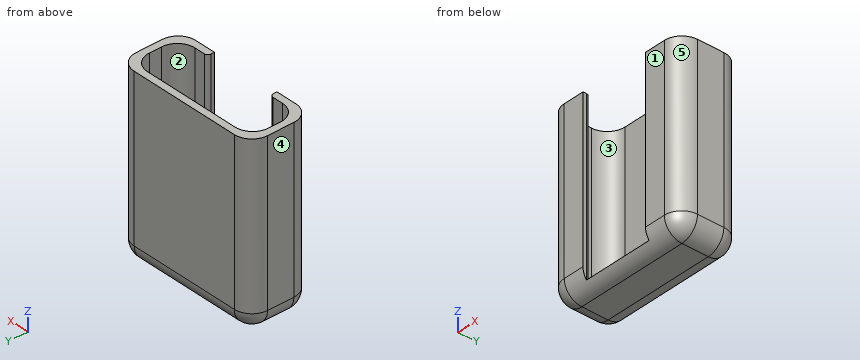
```python
from build123d import *

# Parameters (mm, degrees)
F1_DEPTH     = 50
F0_W         = 20
F0_H         = 2
F2_DEPTH     = 2
F3_T1_DEPTH  = 48
F3_T3_DEPTH  = 57.5
F3_T5_DEPTH  = 32
F3_T7_DEPTH  = 7.5
F3_S11_W     = 5
F3_S11_H     = 5
F3_T12_DEPTH = 5
F3_S17_W     = 5
F3_S17_H     = 5
F3_T18_DEPTH = 5
F3_S23_W     = 5
F3_S23_H     = 5
F3_T24_DEPTH = 5
F3_S29_W     = 5
F3_S29_H     = 5
F3_T30_DEPTH = 5
F4_R         = 1


# Not quite as in the source:
# - a fillet or chamfer that OpenCascade refuses, or shapes differently, is made with other operations: its cross-section is extruded or revolved along the edge and cut away or added


with BuildPart() as f1:
    # F0 (on Top) → F1 (new body)
    with BuildSketch(Plane.XY):
        Polygon((0, 0), (-9, 0), (-9, 13.5), (29, 13.5), (29, 0), (20, 0), (20, -2), (31, -2), (31, 15.5), (-11, 15.5), (-11, -2), (0, -2), align=None)
    extrude(amount=F1_DEPTH)

    # F0 (on Top) → F2 (join)
    with BuildSketch(Plane.XY):
        Polygon((-9, 13.5), (-9, 0), (0, 0), (20, 0), (29, 0), (29, 13.5), align=None)
        with Locations((10, -1)):
            Rectangle(F0_W, F0_H)
    extrude(amount=F2_DEPTH)

    # F3: fillet of radius 5 on 12 edges, made by hand

    # F3_s2 → F3_t1 (join)
    with BuildSketch(Plane.XY.offset(2)):
        with BuildLine():
            ThreePointArc((24, 0), (27.5355339059, 1.4644660941), (29, 5))
            Line((29, 5), (29, 0))
            Line((29, 0), (24, 0))
        make_face()
        with BuildLine():
            ThreePointArc((29, 8.5), (27.5355339059, 12.0355339059), (24, 13.5))
            Line((24, 13.5), (29, 13.5))
            Line((29, 13.5), (29, 8.5))
        make_face()
        with BuildLine():
            ThreePointArc((-4, 0), (-7.5355339059, 1.4644660941), (-9, 5))
            Line((-9, 5), (-9, 0))
            Line((-9, 0), (-4, 0))
        make_face()
        with BuildLine():
            ThreePointArc((-4, 13.5), (-7.5355339059, 12.0355339059), (-9, 8.5))
            Line((-9, 8.5), (-9, 13.5))
            Line((-9, 13.5), (-4, 13.5))
        make_face()
    extrude(amount=F3_T1_DEPTH)

    # F3_s4 → F3_t3 (cut)
    with BuildSketch(Plane.XY.offset(5)):
        with BuildLine():
            ThreePointArc((-6, 15.5), (-9.5355339059, 14.0355339059), (-11, 10.5))
            Line((-11, 10.5), (-11, 15.5))
            Line((-11, 15.5), (-6, 15.5))
        make_face()
        with BuildLine():
            ThreePointArc((-6, -2), (-9.5355339059, -0.5355339059), (-11, 3))
            Line((-11, 3), (-11, -2))
            Line((-11, -2), (-6, -2))
        make_face()
        with BuildLine():
            ThreePointArc((31, 10.5), (29.5355339059, 14.0355339059), (26, 15.5))
            Line((26, 15.5), (31, 15.5))
            Line((31, 15.5), (31, 10.5))
        make_face()
        with BuildLine():
            ThreePointArc((26, -2), (29.5355339059, -0.5355339059), (31, 3))
            Line((31, 3), (31, -2))
            Line((31, -2), (26, -2))
        make_face()
    extrude(amount=F3_T3_DEPTH, mode=Mode.SUBTRACT)

    # F3_s6 → F3_t5 (cut)
    with BuildSketch(Plane.YZ.offset(-6)):
        with BuildLine():
            ThreePointArc((-2, 5), (-0.5355339059, 1.4644660941), (3, 0))
            Line((3, 0), (-2, 0))
            Line((-2, 0), (-2, 5))
        make_face()
        with BuildLine():
            ThreePointArc((15.5, 5), (14.0355339059, 1.4644660941), (10.5, 0))
            Line((10.5, 0), (15.5, 0))
            Line((15.5, 0), (15.5, 5))
        make_face()
    extrude(amount=F3_T5_DEPTH, mode=Mode.SUBTRACT)

    # F3_s8 → F3_t7 (cut)
    with BuildSketch(Plane.XZ.offset(-10.5)):
        with BuildLine():
            ThreePointArc((31, 5), (29.5355339059, 1.4644660941), (26, 0))
            Line((26, 0), (31, 0))
            Line((31, 0), (31, 5))
        make_face()
        with BuildLine():
            ThreePointArc((-11, 5), (-9.5355339059, 1.4644660941), (-6, 0))
            Line((-6, 0), (-11, 0))
            Line((-11, 0), (-11, 5))
        make_face()
    extrude(amount=F3_T7_DEPTH, mode=Mode.SUBTRACT)


with BuildPart() as f3_tool10:
    # F3_s11 → F3_t12 (new body)
    with BuildSketch(Plane.XY.offset(5)):
        with Locations((-8.5, 13)):
            Rectangle(F3_S11_W, F3_S11_H)
    extrude(amount=-F3_T12_DEPTH)

    # F3_s13 → F3_t14 (revolve, cut)
    with BuildSketch(Plane(origin=(-6, 10.5, 5), x_dir=(0.7071067812, -0.7071067812, 0), z_dir=(0.7071067812, 0.7071067812, 0))):
        with BuildLine():
            ThreePointArc((0, -5), (5, 0), (0, 5))
            Line((0, 5), (0, -5))
        make_face()
    revolve(axis=Axis((-6, 10.5, 5), (0, 0, -1)), mode=Mode.SUBTRACT)


with BuildPart() as f1_1:
    add(f1.part)

    # F3_t9: cut F3_tool10
    add(f3_tool10.part, mode=Mode.SUBTRACT)


with BuildPart() as f3_tool16:
    # F3_s17 → F3_t18 (new body)
    with BuildSketch(Plane.XY.offset(5)):
        with Locations((-8.5, 0.5)):
            Rectangle(F3_S17_W, F3_S17_H)
    extrude(amount=-F3_T18_DEPTH)

    # F3_s19 → F3_t20 (revolve, cut)
    with BuildSketch(Plane(origin=(-6, 3, 5), x_dir=(0.7071067812, 0.7071067812, 0), z_dir=(-0.7071067812, 0.7071067812, 0))):
        with BuildLine():
            ThreePointArc((0, -5), (5, 0), (0, 5))
            Line((0, 5), (0, -5))
        make_face()
    revolve(axis=Axis((-6, 3, 5), (0, 0, -1)), mode=Mode.SUBTRACT)


with BuildPart() as f1_2:
    add(f1_1.part)

    # F3_t15: cut F3_tool16
    add(f3_tool16.part, mode=Mode.SUBTRACT)


with BuildPart() as f3_tool22:
    # F3_s23 → F3_t24 (new body)
    with BuildSketch(Plane.XY.offset(5)):
        with Locations((28.5, 13)):
            Rectangle(F3_S23_W, F3_S23_H)
    extrude(amount=-F3_T24_DEPTH)

    # F3_s25 → F3_t26 (revolve, cut)
    with BuildSketch(Plane(origin=(26, 10.5, 5), x_dir=(-0.7071067812, -0.7071067812, 0), z_dir=(0.7071067812, -0.7071067812, 0))):
        with BuildLine():
            ThreePointArc((0, -5), (5, 0), (0, 5))
            Line((0, 5), (0, -5))
        make_face()
    revolve(axis=Axis((26, 10.5, 5), (0, 0, -1)), mode=Mode.SUBTRACT)


with BuildPart() as f1_3:
    add(f1_2.part)

    # F3_t21: cut F3_tool22
    add(f3_tool22.part, mode=Mode.SUBTRACT)


with BuildPart() as f3_tool28:
    # F3_s29 → F3_t30 (new body)
    with BuildSketch(Plane.XY.offset(5)):
        with Locations((28.5, 0.5)):
            Rectangle(F3_S29_W, F3_S29_H)
    extrude(amount=-F3_T30_DEPTH)

    # F3_s31 → F3_t32 (revolve, cut)
    with BuildSketch(Plane(origin=(26, 3, 5), x_dir=(-0.7071067812, 0.7071067812, 0), z_dir=(-0.7071067812, -0.7071067812, 0))):
        with BuildLine():
            ThreePointArc((0, -5), (5, 0), (0, 5))
            Line((0, 5), (0, -5))
        make_face()
    revolve(axis=Axis((26, 3, 5), (0, 0, -1)), mode=Mode.SUBTRACT)


with BuildPart() as f1_4:
    add(f1_3.part)

    # F3_t27: cut F3_tool28
    add(f3_tool28.part, mode=Mode.SUBTRACT)

    # F4
    f4_edges = [f1_4.edges().sort_by_distance(p)[0] for p in [
        (0, 0, 26),
        (20, 0, 26),
    ]]
    fillet(f4_edges, radius=F4_R)


solid = f1_4.part
```
Input: part model. Units: mm. Frame: model coordinates. Face numbers are marked on the shaded views. A direction names the side the tool comes from. Give positions to 0.01 mm unless a question says otherwise; leave off trailing zeros. Loops run counter-clockwise (first coordinate to the right, second up) from the corner with the lowest first, then second, coordinate; pieces in that order, holes last.
1) Contact query for flat-ended pins moving along their axis: pin 1 (0.8 mm diameter, centred on y = -1.5, z = 14.5, fed in from -X); pin 2 (1.5 mm diameter, centred on y = 0.5, z = 10, fed in from +X); pin 3 (1.5 mm diameter, centred on y = 0.5, z = 14, fed in from -X). Output: stop coordinate, or through.
A:
pin 1: stops at x = -8.86
pin 2: stops at x = 30.68
pin 3: stops at x = -10.68
2) Section query D-D on x = 22. Return the cut outline in (y, z), and give its area (3 significant figures).
A:
outline: (-2, 5) arc R5 ccw to (3, 0) - (10.5, 0) arc R5 ccw to (15.5, 5) - (15.5, 50) - (13.5, 50) - (13.5, 2) - (0, 2) - (0, 50) - (-2, 50) - close
area: 216 mm2
3) Reachability of the marked faces 1 and 2 from +Z, -Z, +X, -X, +Y, -Y: full face, straight path, thin tool, end or side. Return the list, or none.
A:
face 1: +Z, -Z, +X, -X, -Y
face 2: +Z
4) Line query: L1, parallel to Y at x = -3, z = 7; L2, parallel to Z at x = -2, y = 6; L3, parallel to Y at x = 4, z = 33. Output: solid intervals per line, ascending.
A:
L1: y = -2 to 0, 13.5 to 15.5
L2: z = 0 to 2
L3: y = 13.5 to 15.5
5) Mould query, pull axis X, two halves, no side actions, for the marked faces 3, 4 and 5. Classes: released by +X, released by -X, zero draft, split by the parting line, or undercut.
A:
face 3: undercut
face 4: released by -X
face 5: released by +X
6) Section query A-A on x = 3.5. Return the cut outline in (y, z).
A:
outline: (-1, 2) arc R5 ccw to (3, 0) - (10.5, 0) arc R5 ccw to (15.5, 5) - (15.5, 50) - (13.5, 50) - (13.5, 2) - close
7) Section query B-B on z = 39.5. Return the cut outline in (x, y).
A:
outline: (-11, 3) arc R5 ccw to (-6, -2) - (0, -2) - (0, -1) arc R1 ccw to (-1, 0) - (-4, 0) arc R5 cw to (-9, 5) - (-9, 8.5) arc R5 cw to (-4, 13.5) - (24, 13.5) arc R5 cw to (29, 8.5) - (29, 5) arc R5 cw to (24, 0) - (21, 0) arc R1 ccw to (20, -1) - (20, -2) - (26, -2) arc R5 ccw to (31, 3) - (31, 10.5) arc R5 ccw to (26, 15.5) - (-6, 15.5) arc R5 ccw to (-11, 10.5) - close
8) Section query C-C on y = 11.75. Return the cut outline in (x, z).
A:
outline: (-10.84, 5) arc R4.84 ccw to (-6, 0.16) - (26, 0.16) arc R4.84 ccw to (30.84, 5) - (30.84, 50) - (27.8, 50) - (27.8, 2) - (-7.8, 2) - (-7.8, 50) - (-10.84, 50) - close
